The model under review builds one solid part; all positions refer to its coordinate system, in mm. Face numbers are marked on the shaded views. Round coordinates to 2 decimals unless told otherwise and drop trailing zeros. Write each loop counter-clockwise with the first axis right and the second up, starting at its lowest first coordinate (ties: lowest second). Pieces come first, ordered by that corner, then holes. Notation, with made-up numbers: M -29.5,-36.75 L 8.5,-36.75 A25 ccw 8.5,-12.75 Z; hole C -9,-24 d11. An arc over 180 degrees is marked long. One line per item, written item: value. Start each with the question number.
1) Mouldability with a two-part tool opening along Z and no side actions: class the marked faces 1, 2, 3 and 4 as +Z half, -Z half, draft (parallel to the pull), parting line (faces both ways), or undercut.
2) Wall thickness on probe 1 along Z at (x, y) = (4.5, 0.35) (3 decimals); probe 2 along Y at (x, z) = (5, -0.15); probe 3 along Y at (x, z) = (6, -1.4): over which ranges is each line inside the solid? List them lowest first.
3) Take a section at B-B, the plane z = -2.3. Write out the cut boundary in (x, y), and give its area (3 significant figures).
4) Take a section at C-C, the plane x = 4.5. Write out the cut boundary in (y, z) (3 decimals).
5) Take a section at A-A, the plane y = 0.4. Write out the cut boundary in (x, z) (3 decimals).
6) For P1, Ø0.6, axis at x = 3.5, y = 0, coming from the +Z side; P2, Ø0.8, axis at x = 4.5, z = -1.5, coming from the -Y side, all flat-tipped, find the tip position at first contact; note any pin that passes through.
from build123d import *

# Parameters (mm, degrees)
SKETCH1_W          = 8.91
SKETCH1_H          = 3.65
MAIN_SHAPE_DEPTH   = 2.65
SKETCH2_W          = 8.41
SKETCH2_H          = 3.15
BOTTOM_BASE_DEPTH  = 0.25
SWITCH_HOLE_W      = 3.91
SWITCH_HOLE_H      = 1.7
CUT_EXTRUDE1_DEPTH = 0.5


with BuildPart() as part:
    # Sketch1 → main shape (new body)
    with BuildSketch(Plane(origin=(0, 0, 0), x_dir=(1, 0, 0), z_dir=(0, 1, 0))):
        with Locations((4.455, 1.825)):
            Rectangle(SKETCH1_W, SKETCH1_H)
    extrude(amount=MAIN_SHAPE_DEPTH)

    # Sketch2 → bottom base (add)
    with BuildSketch(Plane(origin=(0, 2.65, 0), x_dir=(1, 0, 0), z_dir=(0, 1, 0))):
        with Locations((4.455, 1.825)):
            Rectangle(SKETCH2_W, SKETCH2_H)
    extrude(amount=BOTTOM_BASE_DEPTH)

    # switch hole → Cut-Extrude1 (cut)
    with BuildSketch(Plane.XZ):
        with Locations((4.455, -1.825)):
            Rectangle(SWITCH_HOLE_W, SWITCH_HOLE_H)
    extrude(amount=-CUT_EXTRUDE1_DEPTH, mode=Mode.SUBTRACT)


solid = part.part
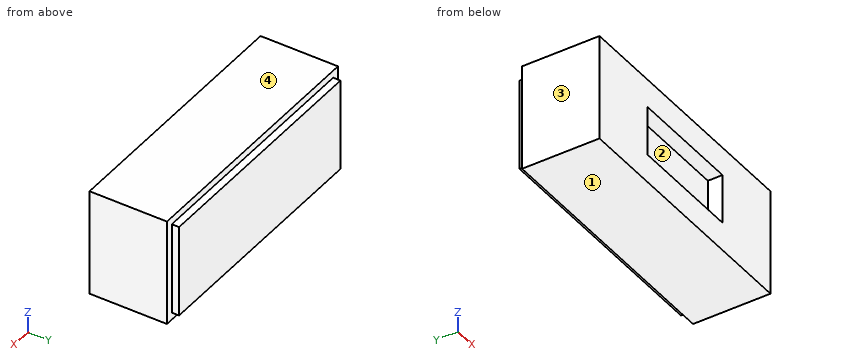
Checked values:
1. face 1: -Z half
1. face 2: undercut
1. face 3: draft
1. face 4: +Z half
2. probe 1: z = -3.65 to -2.675, -0.975 to 0
2. probe 2: y = 0 to 2.65
2. probe 3: y = 0.5 to 2.9
3. outline: M 0,0 L 2.5,0 L 2.5,0.5 L 6.41,0.5 L 6.41,0 L 8.91,0 L 8.91,2.65 L 8.66,2.65 L 8.66,2.9 L 0.25,2.9 L 0.25,2.65 L 0,2.65 Z
3. area: 23.8 mm2
4. outline: M 0,-3.65 L 2.65,-3.65 L 2.65,-3.4 L 2.9,-3.4 L 2.9,-0.25 L 2.65,-0.25 L 2.65,0 L 0,0 L 0,-0.975 L 0.5,-0.975 L 0.5,-2.675 L 0,-2.675 Z
5. outline: M 0,-3.65 L 8.91,-3.65 L 8.91,0 L 0,0 Z; hole M 2.5,-2.675 L 6.41,-2.675 L 6.41,-0.975 L 2.5,-0.975 Z
6. P1: stops at z = 0
6. P2: stops at y = 0.5
